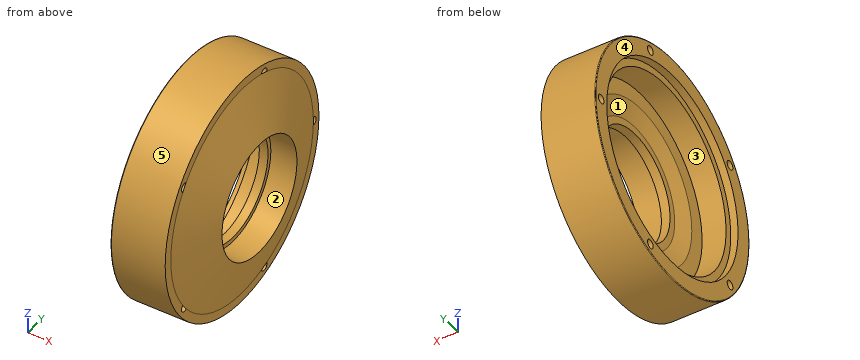
```python
from build123d import *

# Parameters (mm, degrees)
SKETCH2_R          = 6.1
CUT_EXTRUDE1_DEPTH = 74.99773
CIRPATTERN1_COUNT  = 5
FILLET8_R          = 1


with BuildPart() as part:
    # Sketch1 → Revolve1 (revolve)
    with BuildSketch(Plane.XY):
        Polygon((74.997729735, 164), (74.997729735, 152), (98.99091894, 80), (62.997729735, 80), (62.997729735, 74), (50.997729735, 74), (50.997729735, 84), (43, 108), (43, 130), (10, 130), (10, 140), (0, 140), (0, 164), align=None)
    revolve(axis=Axis((0, 0, 0), (1, 0, 0)))

    # Sketch2 → Cut-Extrude1 (cut)
    with BuildSketch(Plane(origin=(74.997729735, 0, 0), x_dir=(0, 0, -1), z_dir=(1, 0, 0))):
        with Locations((0, 152)):
            Circle(SKETCH2_R)
    cut_extrude1 = extrude(amount=-CUT_EXTRUDE1_DEPTH, mode=Mode.SUBTRACT)

    # CirPattern1: Cut-Extrude1 ×5 about axis
    cirpattern1_axis = Axis((0, 0, 0), (1, 0, 0))
    for i in range(1, CIRPATTERN1_COUNT):
        add(cut_extrude1.rotate(cirpattern1_axis, i * 360 / CIRPATTERN1_COUNT), mode=Mode.SUBTRACT)

    # Fillet8
    fillet8_edges = [part.edges().sort_by_distance(p)[0] for p in [
        (0, -164, 0),
    ]]
    fillet(fillet8_edges, radius=FILLET8_R)


solid = part.part
```
The listing builds one solid part. Answer for the finished solid, in the listing's coordinates (mm). Face numbers are marked on the shaded views. A direction names the side the tool comes from. Round coordinates to 2 decimals unless told otherwise and drop trailing zeros. Order: outer loops, then holes, each group sorted by start corner. A loop starts at its lowest first (then second) coordinate and runs counter-clockwise, first axis right, second up. Notation, with made-up numbers: (15, 60.25) - (37, 60.25) arc R32 cw to (37, 87.25) - close; hole circle Ø4 at (50, -26). An arc over 180 degrees is marked (long way). Put each result on its own line as item: value. Start each with the question number.
(1) Find section A-A (y = 0). Give the vertices of the cut face in (x, z), plus the area to 3 significant figures.
(2) Straight lines are drawn through the part: probe 1 along Y at (x, z) = (42.5, 2); probe 2 along Z at (x, y) = (59.5, 49); probe 3 along Z at (x, y) = (3, 0). For each, find the intervals that lie inside material, in ascending order. Write a range as from..to.
(3) For the marked faces 1 and 2, determine the directions among +Z, -Z, +X, -X, +Y, -Y from which every point of the face is accessible in a straight line to the end or side of a thin tool.
(4) Given P1, Ø2, axis at x = 51, y = 126.5, coming from the +Z side; P2, Ø1.5, axis at y = -0.5, z = -102, coming from the +X side; P3, Ø10, axis at x = 39, z = 103, coming from the -Y side, each flat-ended and moving along its own axis, determine where each tip first touches the part or whether it passes through.
(5) Determine the mould class of the marked faces 3, 4 and 5 for opening direction Z: released by +Z, released by -Z, zero draft, split by the parting line, or undercut.
(6) Find section D-D (x = 83.5). Give the vertices of the cut face in (y, z), plus the area to 3 significant figures.
(7) Find section C-C (x = 20). Give the vertices of the cut face in (y, z).
(8) Find section B-B (z = 0). State how many separate pieces and enclosed holes the cut face has, plus the area to 3 significant figures.
Reply:
1. outline: (0, -163) arc R1 ccw to (1, -164) - (75, -164) - (75, -152) - (98.99, -80) - (63, -80) - (63, -74) - (51, -74) - (51, -84) - (43, -108) - (43, -130) - (10, -130) - (10, -140) - (0, -140) - close; (0, 140) - (10, 140) - (10, 130) - (43, 130) - (43, 108) - (51, 84) - (51, 74) - (63, 74) - (63, 80) - (98.99, 80) - (75, 152) - (75, 164) - (1, 164) arc R1 ccw to (0, 163) - close
1. area: 9,710 mm^2
2. probe 1: -163.99..-129.98, 129.98..146.24, 157.76..163.99
2. probe 2: -156.51..-150.31, -138.81..-55.45, 55.45..138.81, 150.31..156.51
2. probe 3: -164..-140, 140..164
3. face 1: -X
3. face 2: +X
4. P1: z = 105.57
4. P2: x = 91.91
4. P3: y = -131.5
5. face 3: undercut
5. face 4: zero draft
5. face 5: split by the parting line
6. outline: circle Ø252.97 at (0, 0); hole circle Ø160 at (0, 0)
6. area: 30,200 mm^2
7. outline: circle Ø328 at (0, 0); hole circle Ø260 at (0, 0); hole circle Ø12.2 at (-122.97, -89.34); hole circle Ø12.2 at (-122.97, 89.34); hole circle Ø12.2 at (46.97, -144.56); hole circle Ø12.2 at (46.97, 144.56); hole circle Ø12.2 at (152, 0)
8. separate pieces: 3
8. enclosed holes: 0
8. area: 8,800 mm^2
